```python
from build123d import *

# Parameters (mm, degrees)
EXTRUDE1_DEPTH         = 12
M10_GEVINDHULLER_D     = 8.5
M10_GEVINDHULLER_DEPTH = 22
M10_GEVINDHULLER_TIP   = 2.553657631


with BuildPart() as part:
    # Sketch1 → Extrude1 (new body)
    with BuildSketch(Plane.XY):
        with BuildLine():
            Line((36.5, 3), (36.5, 5.092922252))
            ThreePointArc((36.5, 5.092922252), (37.855870002, 10.633905611), (41.617082764, 14.922746783))
            Line((41.617082764, 14.922746783), (80.882917236, 42.416980075))
            ThreePointArc((80.882917236, 42.416980075), (84.644129998, 46.705821248), (86, 52.246804607))
            Line((86, 52.246804607), (86, 77))
            ThreePointArc((86, 77), (84.611898825, 79.530174337), (81.732145215, 79.718923361))
            Line((81.732145215, 79.718923361), (11.04340479, 46.756222356))
            ThreePointArc((11.04340479, 46.756222356), (10.379689702, 46.332737476), (9.84900766, 45.751158822))
            ThreePointArc((9.84900766, 45.751158822), (0, 40.60659813), (-9.84900766, 45.751158822))
            ThreePointArc((-9.84900766, 45.751158822), (-10.379689702, 46.332737476), (-11.04340479, 46.756222356))
            Line((-11.04340479, 46.756222356), (-81.732145215, 79.718923361))
            ThreePointArc((-81.732145215, 79.718923361), (-84.611898825, 79.530174337), (-86, 77))
            Line((-86, 77), (-86, 52.246804607))
            ThreePointArc((-86, 52.246804607), (-84.644129998, 46.705821248), (-80.882917236, 42.416980075))
            Line((-80.882917236, 42.416980075), (-41.617082764, 14.922746783))
            ThreePointArc((-41.617082764, 14.922746783), (-37.855870002, 10.633905611), (-36.5, 5.092922252))
            Line((-36.5, 5.092922252), (-36.5, 3))
            ThreePointArc((-36.5, 3), (-35.621320344, 0.878679656), (-33.5, 0))
            Line((-33.5, 0), (0, 0))
            Line((0, 0), (33.5, 0))
            ThreePointArc((33.5, 0), (35.621320344, 0.878679656), (36.5, 3))
        make_face()
    extrude(amount=EXTRUDE1_DEPTH)

    # M10 gevindhuller
    with Locations(Plane.XY.offset(12)):
        with Locations((-59.564002463, 56.141213601), (-36, 45.153138796), (59.564002463, 56.141213601), (36, 45.153138796)):
            Hole(M10_GEVINDHULLER_D / 2, depth=M10_GEVINDHULLER_DEPTH)
            with Locations((0, 0, -(M10_GEVINDHULLER_DEPTH + M10_GEVINDHULLER_TIP / 2))):  # 118° drill point
                Cone(0, M10_GEVINDHULLER_D / 2, M10_GEVINDHULLER_TIP, mode=Mode.SUBTRACT)


solid = part.part
```
Design review of the part built by this model. Coordinates are the model's own, in mm. A direction names the side the tool comes from. Coordinates: 2 decimals unless noted, no trailing zeros. Loops run counter-clockwise (first coordinate to the right, second up) from the corner with the lowest first, then second, coordinate; pieces in that order, holes last. Notation, with made-up numbers: (-17, -28.75) - (24, -28.75) arc R20 ccw to (24, 5.25) - close; hole circle Ø7 at (50, 82.5). An arc over 180 degrees is marked (long way). Use CSV: the item, a comma, the result in double quotes. Start each with the question number.
1) The part is to be moulded in two halves that separate along Y. For faces 1 (the cylindrical face through (-37.893, 10.705, 5.916)), 2 (the cylindrical face through (-31.754, 45.34, 5.916)), 3 (the flat face through (-1, 32, 0)), say which applies: +Y half, -Y half, draft (parallel to the pull), parting line (faces both ways), or undercut.
2) Consider section D-D on y = 35.5. Write out the cut boundary in (x, z), then the cut area to 3 significant figures.
3) Wall thickness on L1, parallel to X at y = 59, z = 1; L2, parallel to Y at x = -33.5, z = 11.25; L3, parallel to Y at x = -36, z = 6.75: over which ranges is each line inside the solid? List them lowest first. Write a range as from..to.
4) Consider section B-B on y = 66.5. Write out the cut boundary in (x, z), then the cut area to 3 significant figures.
5) Consider section A-A on z = 5.5. Write out the cut boundary in (x, y), then the cut area to 3 significant figures.
6) Tool access review of faces 4 (the cylindrical face through (-35.64, 0.9, 5.92)), 5 (the flat face through (46.883, 63.468, 5.916)): name each direction out of +Z, -Z, +X, -X, +Y, -Y from which nothing blocks a thin tool from reaching the whole face with its end or side.
7) Consider section C-C on x = 16. Write out the cut boundary in (y, z), then the cut area to 3 significant figures.
8) For pin 1 Ø1.7 at (y, z) = (4, 8.5) entering from -X; pin 2 Ø11 at (x, y) = (-36, 45.15) entering from +Z; pin 3 Ø2 at (x, z) = (64.5, 10.5) entering from +Y; pin 4 Ø2.5 at (y, z) = (4, 6) entering from +X, all flat-tipped, find the tip position at first contact; note any pin that passes through.
Geometry says:
1,face 1,"-Y half"
1,face 2,"undercut"
1,face 3,"draft"
2,outline,"(-71, 0) - (71, 0) - (71, 12) - (-71, 12) - close"
2,area,"1,700 mm^2"
3,L1,"-86..-62.71, -56.42..-37.3, 37.3..56.42, 62.71..86"
3,L2,"0..41.72, 48.59..57.23"
3,L3,"1.34..40.9, 49.4..58.39"
4,outline,"(-86, 0) - (-53.38, 0) - (-53.38, 12) - (-86, 12) - close; (53.38, 0) - (86, 0) - (86, 12) - (53.38, 12) - close"
4,area,"783 mm^2"
5,outline,"(-86, 52.25) arc R12 ccw to (-80.88, 42.42) - (-41.62, 14.92) arc R12 cw to (-36.5, 5.09) - (-36.5, 3) arc R3 ccw to (-33.5, 0) - (33.5, 0) arc R3 ccw to (36.5, 3) - (36.5, 5.09) arc R12 cw to (41.62, 14.92) - (80.88, 42.42) arc R12 ccw to (86, 52.25) - (86, 77) arc R3 ccw to (81.73, 79.72) - (11.04, 46.76) arc R3 ccw to (9.85, 45.75) arc R12 cw to (-9.85, 45.75) arc R3 ccw to (-11.04, 46.76) - (-81.73, 79.72) arc R3 ccw to (-86, 77) - close; hole circle Ø8.5 at (-59.56, 56.14); hole circle Ø8.5 at (-36, 45.15); hole circle Ø8.5 at (36, 45.15); hole circle Ø8.5 at (59.56, 56.14)"
5,area,"7,490 mm^2"
6,face 4,"+Z, -Z, -X, -Y"
6,face 5,"+Z, -Z, +Y"
7,outline,"(0, 0) - (49.07, 0) - (49.07, 12) - (0, 12) - close"
7,area,"589 mm^2"
8,pin 1,"x = -36.5"
8,pin 2,"z = 12"
8,pin 3,"y = 72.15"
8,pin 4,"x = 36.5"
